Autodesk Fusion 360 part; units mm, degrees
sketch "スケッチ1" plane through (0, 0, 0) normal (0, 0, 1) x (1, 0, 0)
  line L0 (-15.5, 115) -> (-74.5, 115)
  line L1 (-74.5, 115) -> (-74.5, -115)
  line L2 (-74.5, -115) -> (-15.5, -115)
  line L3 (74.5, -5) -> (74.5, 105)
  line L4 (68.0217, 105) -> (-74.5, -115) construction
  line L5 (-74.5, 115) -> (39.1174, -60.3826) construction
  line L6 (-15.5, 115) -> (-15.5, 105)
  line L7 (-15.5, 105) -> (74.5, 105)
  line L8 (-74.5, -115) -> (-15.5, -115) construction
  line L9 (74.5, -25) -> (-15.5, -115)
  line L10 (74.5, -25) -> (-15.5, -25)
  line L11 (-15.5, -25) -> (-15.5, -5)
  line L12 (-15.5, -5) -> (74.5, -5)
  dimension "d2" = 230
  dimension "d5" = 59
  dimension "d7" = 90
  dimension "d8" = 20
extrude "押し出し1" add sketch "スケッチ1" along normal blind 6
chamfer "面取り1" distance 20 angle 45 2 edges at (-74.5, -115, 3) (-74.5, 115, 3)
sketch "スケッチ2" plane through (0, 0, 6) normal (0, 0, 1) x (-1, 0, 0)
  line L0 (54.5, -115) -> (74.5, -95)
  line L1 (74.5, -95) -> (74.5, 95)
  line L2 (74.5, 95) -> (54.5, 115)
  line L3 (54.5, 115) -> (15.5, 115)
  line L4 (15.5, 115) -> (-74.5, 25)
  line L5 (-74.5, 25) -> (15.5, 25)
  line L6 (15.5, 25) -> (15.5, 5)
  line L7 (15.5, 5) -> (-74.5, 5)
  line L8 (-74.5, 5) -> (-74.5, -105)
  line L9 (-74.5, -105) -> (15.5, -105)
  line L10 (15.5, -105) -> (15.5, -115)
  line L11 (15.5, -115) -> (54.5, -115)
  line L12 (-74.5, -105) -> (-34.5, -105) construction
  line L13 (-34.5, -105) -> (-34.5, -75) construction
  line L14 (-34.5, -75) -> (-74.5, -75) construction
  line L15 (-74.5, -75) -> (-74.5, -105) construction
  line L16 (-34.5, -75) -> (-34.5, -25) construction
  point P0 (-34.5, -75)
  point P1 (-34.5, -25)
  dimension "d12" = 40
  dimension "d13" = 30
  dimension "d14" = 50
hole "穴1" at (34.5, 25, 6) at (34.5, 75, 6) direction (0, 0, -1) diameter 18 end through all
equation "d5 = 20 mm + 39 mm"
The listing builds one solid part. Answer for the finished solid, in the listing's coordinates (mm). A direction names the side the tool comes from. Coordinates: 2 decimals unless noted, no trailing zeros. Loops run counter-clockwise (first coordinate to the right, second up) from the corner with the lowest first, then second, coordinate; pieces in that order, holes last. Notation, with made-up numbers: M 42,-9 L 100,-9 A18 ccw 100,19 Z; hole C 32,56.5 d10. An arc over 180 degrees is marked long. Answer in a Markdown table with one row per item.
1) Which of the six approach directions +Z, -Z, +X, -X, +Y, -Y give full straight-line access (tool end or side, diameter ignored) to faces 4 (the cylindrical face through (26.91, 70.16, 2.96)), 5 (the flat face through (30, -25, 3)), 6 (the flat face through (29, 105, 3))?
Answers below:
| item | result |
|---|---|
| face 4 | +Z, -Z |
| face 5 | +Z, -Z, +X |
| face 6 | +Z, -Z, +X, +Y |
2) Find section A-A (x = 34.5). Determine the outline of the cut face in (y, z).
Answers below:
| item | result |
|---|---|
| outline | M -65,0 L -25,0 L -25,6 L -65,6 Z; M -5,0 L 16,0 L 16,6 L -5,6 Z; M 34,0 L 66,0 L 66,6 L 34,6 Z; M 84,0 L 105,0 L 105,6 L 84,6 Z |
3) Find section C-C (z = 4.9). Determine the outline of the cut face in (x, y).
Answers below:
| item | result |
|---|---|
| outline | M -74.5,-95 L -54.5,-115 L -15.5,-115 L 74.5,-25 L -15.5,-25 L -15.5,-5 L 74.5,-5 L 74.5,105 L -15.5,105 L -15.5,115 L -54.5,115 L -74.5,95 Z; hole C 34.5,25 d18; hole C 34.5,75 d18 |
4) Given pin 1 (1.8 mm diameter, centred on x = 38, z = 4, fed in from +Y); pin 2 (11 mm diameter, centred on x = 34.5, y = 25, fed in from -Z); pin 3 (1.8 mm diameter, centred on x = 36, z = 4.5, fed in from -Y); pin 4 (3 mm diameter, centred on y = 111, z = 2, fed in from +X), each flat-ended and moving along its own axis, determine where each tip first touches the part or whether it passes through.
Answers below:
| item | result |
|---|---|
| pin 1 | y = 105 |
| pin 2 | through |
| pin 3 | y = -64.4 |
| pin 4 | x = -15.5 |
5) Find section D-D (y = -41.5). Determine the outline of the cut face in (x, z).
Answers below:
| item | result |
|---|---|
| outline | M -74.5,0 L 58,0 L 58,6 L -74.5,6 Z |
6) Find the intervals of material crossed by probe 1 along X at (y, z) = (25, 2.4); probe 2 along X at (y, z) = (-18, 0.55); probe 3 along Y at (x, z) = (56.5, 3.4), in increasing order.
Answers below:
| item | result |
|---|---|
| probe 1 | -74.5 to 25.5, 43.5 to 74.5 |
| probe 2 | -74.5 to -15.5 |
| probe 3 | -43 to -25, -5 to 105 |
7) Find section B-B (y = 25). Determine the outline of the cut face in (x, z), then the cut area to 3 significant figures.
Answers below:
| item | result |
|---|---|
| outline | M -74.5,0 L 25.5,0 L 25.5,6 L -74.5,6 Z; M 43.5,0 L 74.5,0 L 74.5,6 L 43.5,6 Z |
| area | 786 mm^2 |
8) Determine the mould class of faces 1 (the flat face through (-35, 115, 3)), 2 (the flat face through (-18, 2, 0)), 3 (the cylindrical face through (26.91, 20.16, 2.96)) for opening direction Y: released by +Y, released by -Y, zero draft, split by the parting line, or undercut.
Answers below:
| item | result |
|---|---|
| face 1 | released by +Y |
| face 2 | zero draft |
| face 3 | undercut |
